Work out the finished part from the listing and answer in its coordinate system (mm). Coordinates: 2 decimals unless noted, no trailing zeros. Order: outer loops, then holes, each group sorted by start corner. A loop starts at its lowest first (then second) coordinate and runs counter-clockwise, first axis right, second up. Notation, with made-up numbers: M -1.5,60 L 28.5,60 A13 ccw 28.5,72 Z; hole C 32,-2 d3. An arc over 180 degrees is marked long. Write item = value, one per line. Start each with the question number.
Q1. Find section A-A on y = 0. Give the vertices of the cut face in (x, z), and give its area (3 significant figures).
Q2. Find section C-C on z = 3.75. Give the vertices of the cut face in (x, y), and give its area (3 significant figures).
Q3. Straight lines are drawn through the part: line 1 along Y through (x, z) = (70, 5.75); line 2 along X through (y, z) = (-95, 2.5); line 3 along Y through (x, z) = (0, 2.5). For each, find the intervals that lie inside material, in ascending order.
Q4. Find section B-B on x = 0. Give the vertices of the cut face in (y, z).
Q5. Each of these flat-tipped pins is pushed along its axis until it touches: P1, Ø5.5, axis at x = -70, y = -95, coming from the -Z side; P2, Ø8, axis at x = 70, y = 95, coming from the -Z side (3 decimals). Where does it stop, or does it pass through?
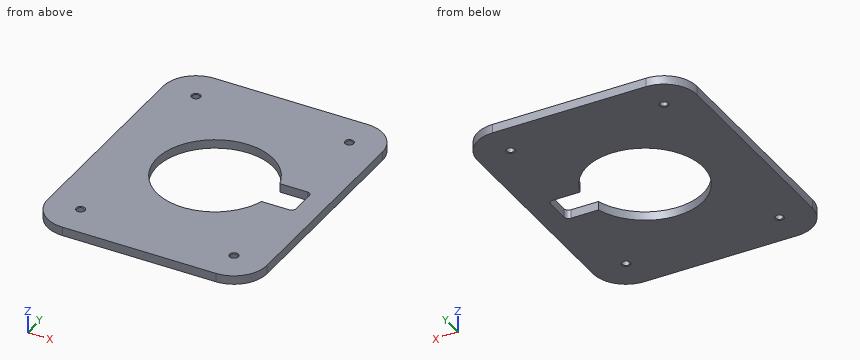
```python
from build123d import *

# Parameters (mm, degrees)
SKIZZE1_W                       = 200
SKIZZE1_H                       = 250
AUFSATZ_LINEAR_AUSTRAGEN1_DEPTH = 8
VERRUNDUNG1_R                   = 30
VERRUNDUNG2_R                   = 4
M8_GEWINDEBOHRUNG1_AT_2_COUNT   = 2
M8_GEWINDEBOHRUNG1_AT_2_PITCH   = 140
M8_GEWINDEBOHRUNG1_AT_3_COUNT   = 2
M8_GEWINDEBOHRUNG1_AT_3_PITCH   = 236.008474424
M8_GEWINDEBOHRUNG1_AT_4_COUNT   = 2
M8_GEWINDEBOHRUNG1_AT_4_PITCH   = 190


with BuildPart() as part:
    # Skizze1 → Aufsatz-Linear austragen1 (new body)
    with BuildSketch(Plane.XY):
        Rectangle(SKIZZE1_W, SKIZZE1_H)
        with BuildLine():
            Line((50.833060109, 15), (80, 15))
            Line((80, 15), (80, -15))
            Line((80, -15), (50.833060109, -15))
            ThreePointArc((50.833060109, -15), (-53, 0), (50.833060109, 15))
        make_face(mode=Mode.SUBTRACT)
    extrude(amount=AUFSATZ_LINEAR_AUSTRAGEN1_DEPTH)

    # Verrundung1
    verrundung1_edges = [part.edges().sort_by_distance(p)[0] for p in [
        (100, -125, 4),
        (-100, -125, 4),
        (-100, 125, 4),
        (100, 125, 4),
    ]]
    fillet(verrundung1_edges, radius=VERRUNDUNG1_R)

    # Verrundung2
    verrundung2_edges = [part.edges().sort_by_distance(p)[0] for p in [
        (80, -15, 4),
        (80, 15, 4),
    ]]
    fillet(verrundung2_edges, radius=VERRUNDUNG2_R)

    # Skizze3 → M8 Gewindebohrung1 (revolve, cut)
    with BuildSketch(Plane(origin=(70, 95, 0), x_dir=(0, 1, 0), z_dir=(1, 0, 0))):
        Polygon((0, 0), (0, 8), (4.025, 8), (3.4, 7.375), (3.4, 0.625), (4.025, 0), align=None)
    m8_gewindebohrung1 = revolve(axis=Axis((70, 95, -6.35), (0, 0, 1)), mode=Mode.SUBTRACT)

    # M8 Gewindebohrung1 at 2: M8 Gewindebohrung1 ×2
    with Locations(*[(-i * M8_GEWINDEBOHRUNG1_AT_2_PITCH, 0, 0) for i in range(1, M8_GEWINDEBOHRUNG1_AT_2_COUNT)]):
        add(m8_gewindebohrung1, mode=Mode.SUBTRACT)

    # M8 Gewindebohrung1 at 3: M8 Gewindebohrung1 ×2
    with Locations(*[Vector(-0.593199038, -0.805055837, 0) * (i * M8_GEWINDEBOHRUNG1_AT_3_PITCH) for i in range(1, M8_GEWINDEBOHRUNG1_AT_3_COUNT)]):
        add(m8_gewindebohrung1, mode=Mode.SUBTRACT)

    # M8 Gewindebohrung1 at 4: M8 Gewindebohrung1 ×2
    with Locations(*[(0, -i * M8_GEWINDEBOHRUNG1_AT_4_PITCH, 0) for i in range(1, M8_GEWINDEBOHRUNG1_AT_4_COUNT)]):
        add(m8_gewindebohrung1, mode=Mode.SUBTRACT)


solid = part.part
```
Findings below:
q1.outline = M -100,0 L -53,0 L -53,8 L -100,8 Z; M 80,0 L 100,0 L 100,8 L 80,8 Z
q1.area = 536 mm^2
q2.outline = M -100,-95 A30 ccw -70,-125 L 70,-125 A30 ccw 100,-95 L 100,95 A30 ccw 70,125 L -70,125 A30 ccw -100,95 Z; hole C -70,-95 d6.8; hole C -70,95 d6.8; hole M 50.83,-15 L 76,-15 A4 ccw 80,-11 L 80,11 A4 ccw 76,15 L 50.83,15 A53 ccw long Z; hole C 70,-95 d6.8; hole C 70,95 d6.8
q2.area = 39,400 mm^2
q3.line_1 = -125 to -98.4, -91.6 to -15, 15 to 91.6, 98.4 to 125
q3.line_2 = -100 to -73.4, -66.6 to 66.6, 73.4 to 100
q3.line_3 = -125 to -53, 53 to 125
q4.outline = M -125,0 L -53,0 L -53,8 L -125,8 Z; M 53,0 L 125,0 L 125,8 L 53,8 Z
q5.P1 = through
q5.P2 = 0.025
